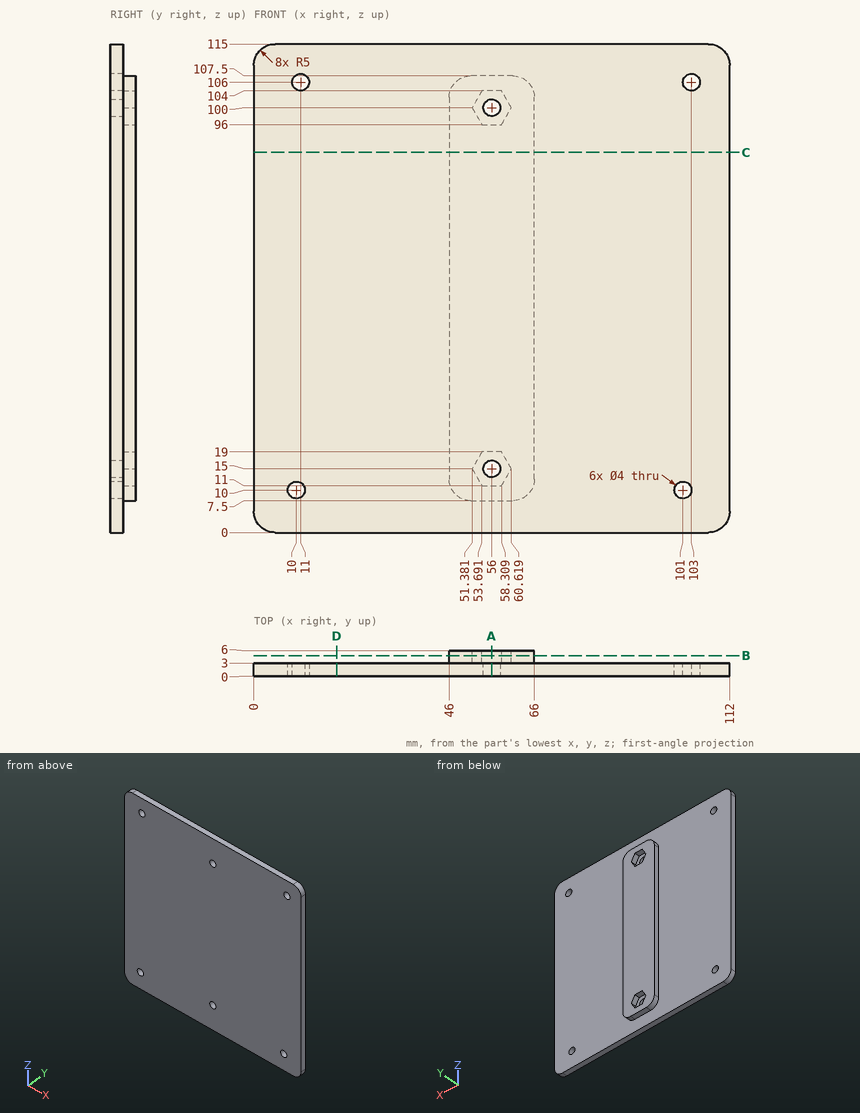
The drawing under review shows one solid part. Ordinate dimensions are in mm from its lowest x, y, z. Round coordinates to 2 decimals unless told otherwise and drop trailing zeros. Write each loop counter-clockwise with the first axis right and the second up, starting at its lowest first coordinate (ties: lowest second). Pieces come first, ordered by that corner, then holes. Notation, with made-up numbers: (8.25, -22) - (58.25, -22) arc R21 ccw to (58.25, -4) - close; hole circle Ø8 at (76.25, 78). An arc over 180 degrees is marked (long way). Write each question's results on one line, items separated by ' | '.
Item 1: Take a section at A-A on x = 56. State the section outline as (y, z) points.
Calculated:
outline: (0, 0) - (3, 0) - (3, 7.5) - (6, 7.5) - (6, 11) - (3, 11) - (3, 13) - (0, 13) - close; (0, 17) - (3, 17) - (3, 19) - (6, 19) - (6, 96) - (3, 96) - (3, 98) - (0, 98) - close; (0, 102) - (3, 102) - (3, 104) - (6, 104) - (6, 107.5) - (3, 107.5) - (3, 115) - (0, 115) - close
Item 2: To check wall thickness, follow line 1 along X through (y, z) = (1.55, 15); line 2 along Z through (x, y) = (56, 0.75); line 3 along Z through (x, y) = (10, 1). State the ranges of each line that lie inside material, in increasing order. Write a range as from..to.
Calculated:
line 1: x = 0..54, 58..112 | line 2: z = 0..13, 17..98, 102..115 | line 3: z = 0..8, 12..104.27, 107.73..115
Item 3: Take a section at B-B on y = 4.8. State the section outline as (x, z) points, then the cut area to 3 significant figures.
Calculated:
outline: (46, 12.5) arc R5 ccw to (51, 7.5) - (61, 7.5) arc R5 ccw to (66, 12.5) - (66, 102.5) arc R5 ccw to (61, 107.5) - (51, 107.5) arc R5 ccw to (46, 102.5) - close; hole (51.38, 15) - (53.69, 11) - (58.31, 11) - (60.62, 15) - (58.31, 19) - (53.69, 19) - close; hole (51.38, 100) - (53.69, 96) - (58.31, 96) - (60.62, 100) - (58.31, 104) - (53.69, 104) - close | area: 1,870 mm^2
Item 4: For pin 1 (5 mm diameter, centred on x = 11, z = 106, fed in from +Y); pin 2 (0.9 mm diameter, centred on x = 58.5, y = 5, fed in from -Z); pin 3 (2.5 mm diameter, centred on y = 4.5, z = 66, fed in from -X), all flat-tipped, find the tip position at first contact; note any pin that passes through.
Calculated:
pin 1: stops at y = 3 | pin 2: stops at z = 7.5 | pin 3: stops at x = 46
Item 5: Take a section at C-C on z = 89.5. State the section outline as (x, y) points, then the cut area to 3 significant figures.
Calculated:
outline: (0, 0) - (112, 0) - (112, 3) - (66, 3) - (66, 6) - (46, 6) - (46, 3) - (0, 3) - close | area: 396 mm^2
Item 6: Take a section at D-D on x = 19.5. State the section outline as (y, z) points.
Calculated:
outline: (0, 0) - (3, 0) - (3, 115) - (0, 115) - close
